Geometry check sheet. Reference: the model listing, model coordinates, mm. Face numbers are marked on the shaded views. A direction names the side the tool comes from. Give positions to 0.01 mm unless a question says otherwise; leave off trailing zeros. Loops run counter-clockwise (first coordinate to the right, second up) from the corner with the lowest first, then second, coordinate; pieces in that order, holes last. Notation, with made-up numbers: (-39, 9.25) -> (2, 9.25) arc R14 ccw to (2, 17.25) -> close; hole circle Ø5 at (58.5, 5.5). An arc over 180 degrees is marked (long way). One line per item, written item: value. Start each with the question number.
(1) Sectioned sample at C-C, the plane z = 41.5. Record the cut outline in (x, y), then the cut area to 3 significant figures.
(2) Sectioned sample at B-B, the plane x = 15.5. Record the cut outline in (y, z).
(3) Scan lines: line 1 along Y through (x, z) = (-24.5, 42.5); line 2 along Z through (x, y) = (4, -21.5); line 3 along Z through (x, y) = (3, -18). Record each from-to range of solid material in increasing order. Write a range as from..to.
(4) Sectioned sample at A-A, the plane z = 32. Record the cut outline in (x, y).
(5) Tool access check on the marked faces 1, 2 and 3. Record the directions out of +Z, -Z, +X, -X, +Y, -Y that give a thin tool (end or side, any length) a straight path to the whole face; none if there is none.
(6) Sectioned sample at D-D, the plane x = -25. Record the cut outline in (y, z).
from build123d import *

# Parameters (mm, degrees)
F0_W     = 56.53508
F0_H     = 59.804362
F1_DEPTH = 50
F3_DEPTH = 15


with BuildPart() as f1:
    # F0 (on Top) → F1 (new body)
    with BuildSketch(Plane.XY):
        Rectangle(F0_W, F0_H)
    extrude(amount=F1_DEPTH)

    # F2 (on face) → F3 (cut)
    with BuildSketch(Plane.XZ.offset(29.902181)):
        with BuildLine():
            ThreePointArc((0, 50), (19.988169, 41.720629), (28.26754, 21.73246))
            Line((28.26754, 21.73246), (28.26754, 50))
            Line((28.26754, 50), (0, 50))
        make_face()
        with BuildLine():
            ThreePointArc((-28.26754, 21.73246), (-19.988169, 41.720629), (0, 50))
            Line((0, 50), (-28.26754, 50))
            Line((-28.26754, 50), (-28.26754, 21.73246))
        make_face()
    extrude(amount=-F3_DEPTH, mode=Mode.SUBTRACT)


solid = f1.part
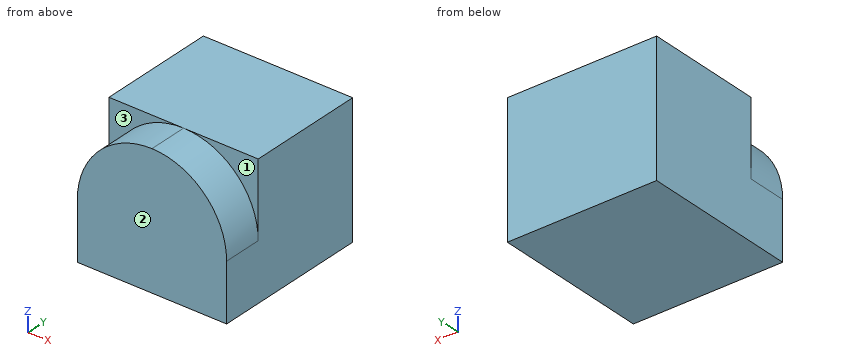
Calculated:
1. outline: (-28.27, -14.9) -> (-20.21, -14.9) -> (-20.21, -29.9) -> (20.21, -29.9) -> (20.21, -14.9) -> (28.27, -14.9) -> (28.27, 29.9) -> (-28.27, 29.9) -> close
1. area: 3,140 mm2
2. outline: (-29.9, 0) -> (29.9, 0) -> (29.9, 50) -> (-14.9, 50) -> (-14.9, 45.37) -> (-29.9, 45.37) -> close
3. line 1: y = -14.9..29.9
3. line 2: z = 0..49.72
3. line 3: z = 0..49.84
4. outline: (-28.27, -14.9) -> (-26.34, -14.9) -> (-26.34, -29.9) -> (26.34, -29.9) -> (26.34, -14.9) -> (28.27, -14.9) -> (28.27, 29.9) -> (-28.27, 29.9) -> close
5. face 1: +Z, +X, -Y
5. face 2: +Z, -Z, +X, -X, -Y
5. face 3: +Z, -X, -Y
6. outline: (-29.9, 0) -> (29.9, 0) -> (29.9, 50) -> (-14.9, 50) -> (-14.9, 34.93) -> (-29.9, 34.93) -> close
